Could you check a few things on this drawing? It's one solid part, dimensions in mm from its lowest x, y, z. Coordinates: 2 decimals unless noted, no trailing zeros. Write each loop counter-clockwise with the first axis right and the second up, starting at its lowest first coordinate (ties: lowest second). Pieces come first, ordered by that corner, then holes.
Item 1: I'm going to push flat-ended pins straight in: P1, Ø6, axis at x = 11, z = 5, coming from the +Y side; P2, Ø7, axis at x = 7.94, y = 75, coming from the -Z side; P3, Ø3, axis at y = 160, z = 6, coming from the +X side. Where does each tip first touch, or does it pass through?
Item 2: I want a section at A-A (z = 4.76). Please give me the cut outline in (x, y).
Item 3: I want a section at B-B (y = 196). Please give me the cut outline in (x, z).
Item 4: Please list where these lines run through material, in increasing order: line 1 (Y direction, x = 7.94, z = 11.95); line 2 (Y direction, x = 0.95, z = 4.76); line 3 (X direction, y = 253.6, z = 11.6).
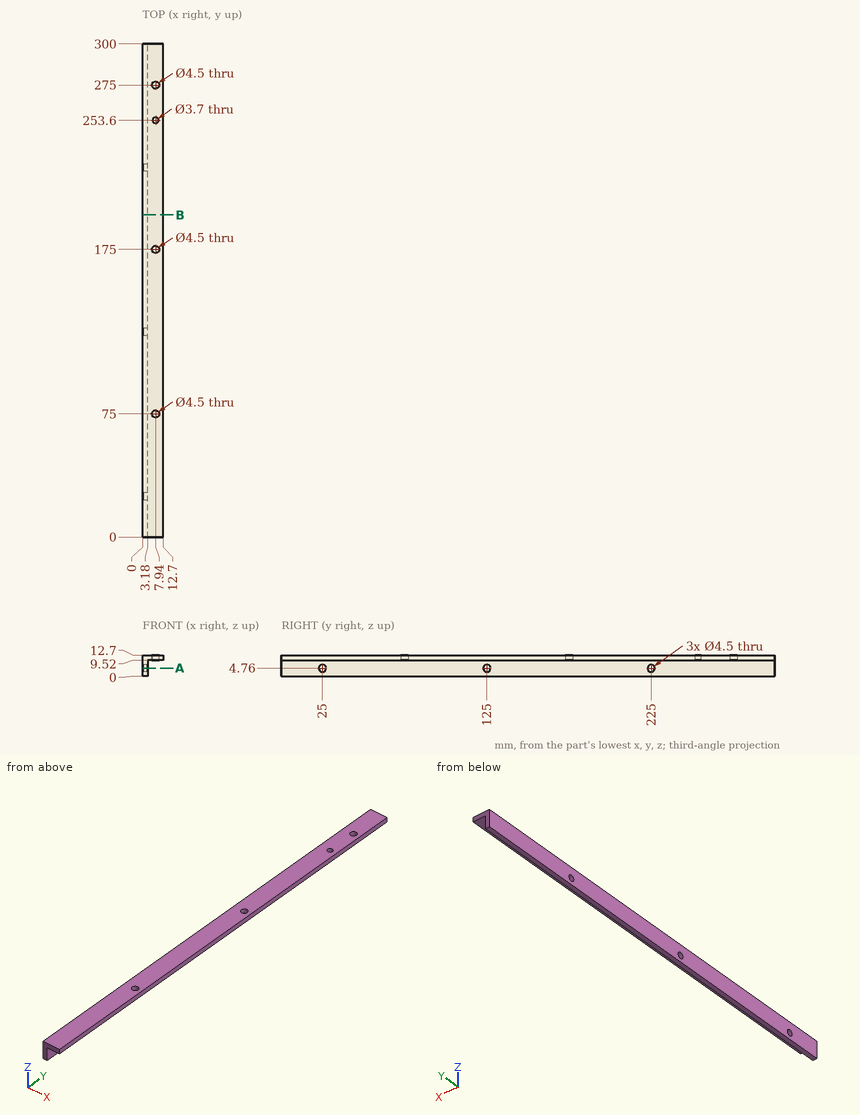
Answer:
1. P1: passes through
1. P2: stops at z = 9.52
1. P3: stops at x = 3.18
2. outline: (0, 0) - (3.18, 0) - (3.18, 22.75) - (0, 22.75) - close; (0, 27.25) - (3.18, 27.25) - (3.18, 122.75) - (0, 122.75) - close; (0, 127.25) - (3.18, 127.25) - (3.18, 222.75) - (0, 222.75) - close; (0, 227.25) - (3.18, 227.25) - (3.18, 300) - (0, 300) - close
3. outline: (0, 0) - (3.18, 0) - (3.18, 9.52) - (12.7, 9.52) - (12.7, 12.7) - (0, 12.7) - close
4. line 1: y = 0 to 72.75, 77.25 to 172.75, 177.25 to 251.75, 255.45 to 272.75, 277.25 to 300
4. line 2: y = 0 to 22.75, 27.25 to 122.75, 127.25 to 222.75, 227.25 to 300
4. line 3: x = 0 to 6.09, 9.79 to 12.7
